Input: part model. Units: mm. Frame: model coordinates. Face numbers are marked on the shaded views. A direction names the side the tool comes from. Round coordinates to 2 decimals unless told otherwise and drop trailing zeros. Order: outer loops, then holes, each group sorted by start corner. A loop starts at its lowest first (then second) coordinate and runs counter-clockwise, first axis right, second up. Notation, with made-up numbers: (-8.75, -25) - (5.25, -25) arc R30 cw to (5.25, 7) - close; hole circle Ø5 at (87.5, 54.25). An arc over 180 degrees is marked (long way). One line per item, written item: value. Start each with the question number.
from build123d import *

# Parameters (mm, degrees)
SKETCH_1_W           = 25
SKETCH_1_H           = 21
EXTRUDE_2_DEPTH      = 34
SKETCH_2_W           = 10
SKETCH_2_H           = 9
SKETCH_2_R           = 1
CUT_EXTRUDE_4_DEPTH  = 60
SKETCH_3_R           = 1
SKETCH_3_W           = 13
SKETCH_3_H           = 38
CUT_EXTRUDE_2_DEPTH  = 44.488504228
SKETCH_6_W           = 3.5
SKETCH_6_H           = 7
CUT_EXTRUDE_5_DEPTH  = 9
SKETCH_11_W          = 3.5
SKETCH_11_H          = 7
CUT_EXTRUDE_9_DEPTH  = 9
SKETCH_7_R           = 1.25
CUT_EXTRUDE_6_DEPTH  = 42.871828238
SKETCH_9_W           = 25
SKETCH_9_H           = 10
CUT_EXTRUDE_7_DEPTH  = 2
SKETCH_10_W          = 25
SKETCH_10_H          = 10
CUT_EXTRUDE_8_DEPTH  = 2
CUT_EXTRUDE_START    = -6
SKETCH_12_W          = 13
SKETCH_12_H          = 68
CUT_EXTRUDE_10_DEPTH = 6
EXTRUDE_4_DEPTH      = 1.5
FILLET_R2_R          = 2
FILLET_R1_R          = 1


with BuildPart() as part:
    # 草图1 → 凸台-拉伸2 (new, symmetric)
    with BuildSketch(Plane(origin=(0, 0, 0), x_dir=(1, 0, 0), z_dir=(0, 1, 0))):
        Rectangle(SKETCH_1_W, SKETCH_1_H)
        Polygon((11.5, -3.5), (11.5, -6.5), (6.5, -6.5), (6, -6.5), (-6, -6.5), (-6.5, -6.5), (-11.5, -6.5), (-11.5, -3.5), (-6.5, -3.5), (-6.5, 3.5), (-11.5, 3.5), (-11.5, 6.5), (-6.5, 6.5), (-6, 6.5), (6, 6.5), (6.5, 6.5), (11.5, 6.5), (11.5, 3.5), (6.5, 3.5), (6.5, -3.5), align=None, mode=Mode.SUBTRACT)
    extrude(amount=EXTRUDE_2_DEPTH, both=True)

    # 草图2 → 切除-拉伸4 (cut)
    with BuildSketch(Plane(origin=(0, 0, -10.5), x_dir=(-1, 0, 0), z_dir=(0, 0, -1))):
        Polygon((9, -15), (9, 15), (6.25, 15), (6.25, 20), (3.25, 20), (3.25, 15), (-3.25, 15), (-3.25, 20), (-6.25, 20), (-6.25, 15), (-9, 15), (-9, -15), (-6.25, -15), (-6.25, -20), (-3.25, -20), (-3.25, -15), (3.25, -15), (3.25, -20), (6.25, -20), (6.25, -15), align=None)
        with Locations((0, -29.5)):
            Rectangle(SKETCH_2_W, SKETCH_2_H)
        with Locations((8.5, -22)):
            Circle(SKETCH_2_R)
        with Locations((-8.5, -22)):
            Circle(SKETCH_2_R)
        with Locations((-8.5, 22)):
            Circle(SKETCH_2_R)
        with Locations((8.5, 22)):
            Circle(SKETCH_2_R)
    extrude(amount=-CUT_EXTRUDE_4_DEPTH, mode=Mode.SUBTRACT)

    # 草图3 → 切除-拉伸2 (cut, through all)
    with BuildSketch(Plane(origin=(12.5, 0, 0), x_dir=(0, 0, -1), z_dir=(1, 0, 0))):
        with Locations((8.5, -17)):
            Circle(SKETCH_3_R)
        with Locations(Location((8.5, 17, 0), (0, 0, 180))):
            Circle(SKETCH_3_R)
        with Locations((-8.5, 17)):
            Circle(SKETCH_3_R)
        with Locations((-8.5, -17)):
            Circle(SKETCH_3_R)
        Rectangle(SKETCH_3_W, SKETCH_3_H)
    extrude(amount=-CUT_EXTRUDE_2_DEPTH, mode=Mode.SUBTRACT)

    # 草图6 → 切除-拉伸5 (cut)
    with BuildSketch(Plane.XZ.offset(34)):
        with Locations((8.25, 0)):
            Rectangle(SKETCH_6_W, SKETCH_6_H)
        with Locations((-8.25, 0)):
            Rectangle(SKETCH_6_W, SKETCH_6_H)
    extrude(amount=-CUT_EXTRUDE_5_DEPTH, mode=Mode.SUBTRACT)

    # 草图11 → 切除-拉伸9 (cut)
    with BuildSketch(Plane(origin=(0, 34, 0), x_dir=(1, 0, 0), z_dir=(0, 1, 0))):
        with Locations((-8.25, 0)):
            Rectangle(SKETCH_11_W, SKETCH_11_H)
        with Locations((8.25, 0)):
            Rectangle(SKETCH_11_W, SKETCH_11_H)
    extrude(amount=-CUT_EXTRUDE_9_DEPTH, mode=Mode.SUBTRACT)

    # 草图7 → 切除-拉伸6 (cut, through all)
    with BuildSketch(Plane(origin=(0, 0, -10.5), x_dir=(-1, 0, 0), z_dir=(0, 0, -1))):
        with Locations((8, -29)):
            Circle(SKETCH_7_R)
        with Locations(Location((-8, -29, 0), (0, 0, 180))):
            Circle(SKETCH_7_R)
        with Locations((-8, 29)):
            Circle(SKETCH_7_R)
        with Locations(Location((8, 29, 0), (0, 0, 180))):
            Circle(SKETCH_7_R)
    extrude(amount=-CUT_EXTRUDE_6_DEPTH, mode=Mode.SUBTRACT)

    # 草图9 → 切除-拉伸7 (cut)
    with BuildSketch(Plane(origin=(0, 0, -10.5), x_dir=(-1, 0, 0), z_dir=(0, 0, -1))):
        with Locations((0, 29)):
            Rectangle(SKETCH_9_W, SKETCH_9_H)
    extrude(amount=-CUT_EXTRUDE_7_DEPTH, mode=Mode.SUBTRACT)

    # 草图10 → 切除-拉伸8 (cut)
    with BuildSketch(Plane.XY.offset(10.5)):
        with Locations((0, 29)):
            Rectangle(SKETCH_10_W, SKETCH_10_H)
    extrude(amount=-CUT_EXTRUDE_8_DEPTH, mode=Mode.SUBTRACT)

    # 草图12 → 切除-拉伸10 (cut)
    with BuildSketch(Plane(origin=(12.5, 0, 0), x_dir=(0, 0, -1), z_dir=(1, 0, 0)).offset(CUT_EXTRUDE_START)):
        Rectangle(SKETCH_12_W, SKETCH_12_H)
    extrude(amount=CUT_EXTRUDE_10_DEPTH, mode=Mode.SUBTRACT)

    # 草图13 → 凸台-拉伸4 (add)
    with BuildSketch(Plane(origin=(-11.5, 0, 0), x_dir=(0, 0, -1), z_dir=(1, 0, 0))):
        with BuildLine():
            Line((-6.5, -34), (-3.5, -34))
            Line((-3.5, -34), (-3.5, -23.5))
            ThreePointArc((-3.5, -23.5), (-5, -25), (-6.5, -23.5))
            Line((-6.5, -23.5), (-6.5, -34))
        make_face()
        with BuildLine():
            Line((3.5, -34), (3.5, -23.5))
            ThreePointArc((3.5, -23.5), (5, -25), (6.5, -23.5))
            Line((6.5, -23.5), (6.5, -34))
            Line((6.5, -34), (3.5, -34))
        make_face()
        with BuildLine():
            Line((-3.5, 34), (-3.5, 23.5))
            ThreePointArc((-3.5, 23.5), (-5, 25), (-6.5, 23.5))
            Line((-6.5, 23.5), (-6.5, 34))
            Line((-6.5, 34), (-3.5, 34))
        make_face()
        with BuildLine():
            Line((6.5, 34), (6.5, 23.5))
            ThreePointArc((6.5, 23.5), (5, 25), (3.5, 23.5))
            Line((3.5, 23.5), (3.5, 34))
            Line((3.5, 34), (6.5, 34))
        make_face()
    extrude(amount=EXTRUDE_4_DEPTH)

    # R2
    fillet_r2_edges = [part.edges().sort_by_distance(p)[0] for p in [
        (5, -25, 8.5),
        (5, -25, -8.5),
        (-5, -25, 8.5),
        (-5, -25, -8.5),
        (9, -15, 8.5),
        (9, -15, -8.5),
        (9, 15, 8.5),
        (9, 15, -8.5),
        (-9, 15, 8.5),
        (-9, 15, -8.5),
        (-9, -15, 8.5),
        (-9, -15, -8.5),
        (-12, -19, 6.5),
        (-12, 19, -6.5),
        (-12, 19, 6.5),
        (-12, -19, -6.5),
    ]]
    fillet(fillet_r2_edges, radius=FILLET_R2_R)

    # R1
    fillet_r1_edges = [part.edges().sort_by_distance(p)[0] for p in [
        (-3.25, -20, 8.5),
        (-3.25, -20, -8.5),
        (-6.25, -20, 8.5),
        (-6.25, -20, -8.5),
        (3.25, -20, 8.5),
        (3.25, -20, -8.5),
        (6.25, -20, 8.5),
        (6.25, -20, -8.5),
        (6.25, 20, 8.5),
        (6.25, 20, -8.5),
        (3.25, 20, 8.5),
        (3.25, 20, -8.5),
        (-3.25, 20, 8.5),
        (-3.25, 20, -8.5),
        (-6.25, 20, 8.5),
        (-6.25, 20, -8.5),
    ]]
    fillet(fillet_r1_edges, radius=FILLET_R1_R)


solid = part.part
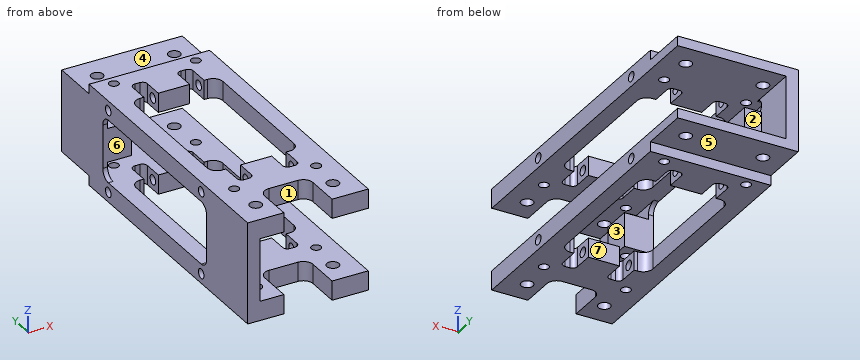
Item 1: First-contact query: pin 1 Ø5 at (y, z) = (-29, 3) entering from +X; pin 2 Ø0.5 at (x, z) = (4.5, 8) entering from -Y; pin 3 Ø4.5 at (x, z) = (1.5, -8.5) entering from -Y. Flat tips, straight axial feed; report the tip coordinate or a pass-through.
Item 2: Section query B-B on y = -29. Give the number of separate pieces and of enclosed holes in the cut face, and give its area (4 significant figures).
Item 3: Section query C-C on z = 2.75. Return loops of the section in (x, y), and give its area (3 significant figures).
Item 4: Reachability of the marked faces 4, 5, 6 and 7 from +Z, -Z, +X, -X, +Y, -Y: full face, straight path, thin tool, end or side. Return the list, or none.
Item 5: Line query: L1, parallel to Z at x = -8, y = 15; L2, parallel to X at y = -2, z = -7.25; L3, parallel to Y at x = -3, z = -9. Output: solid intervals per line, ascending.
Item 6: Section query D-D on y = -6.5. Return loops of the section in (x, z), and give its area (3 significant figures).
Item 7: Section query A-A on x = 10.25. Return loops of the section in (y, z).
Item 8: Pull-direction query (X, two-part tool) for the marked faces 1, 2 and 3; classes: released by +X, released by -X, zero draft, split by the parting line, or undercut.
Geometry results:
1. pin 1: stops at x = -10
1. pin 2: stops at y = -26.03
1. pin 3: stops at y = -25.15
2. separate pieces: 7
2. enclosed holes: 0
2. area: 112.5 mm^2
3. outline: (-12.5, -34) - (-10, -34) - (-10, -25) - (-6.5, -25) - (-6.5, -19) - (-12.5, -19) - close; (-12.5, 19) - (-6.5, 19) - (-6.5, 25) - (-10, 25) - (-10, 34) - (-12.5, 34) - close; hole circle Ø2 at (-8.5, -22); hole circle Ø2 at (-8.5, 22)
3. area: 111 mm^2
4. face 4: +Z, +X, -X, +Y
4. face 5: -Z, +X, -X, +Y
4. face 6: +X, -X
4. face 7: +Z, -Z
5. L1: z = -10.5 to -6.5, 6.5 to 10.5
5. L2: x = -12.5 to -9, 9 to 12.5
5. L3: y = -25 to -17.87, -16.13 to -15, 15 to 16.13, 17.87 to 24
6. outline: (-12.5, -10.5) - (-9, -10.5) - (-9, -6.5) - (-12.5, -6.5) - close; (-12.5, 6.5) - (-9, 6.5) - (-9, 10.5) - (-12.5, 10.5) - close; (9, -10.5) - (12.5, -10.5) - (12.5, -6.5) - (9, -6.5) - close; (9, 6.5) - (12.5, 6.5) - (12.5, 10.5) - (9, 10.5) - close
6. area: 56.0 mm^2
7. outline: (-34, -10.5) - (24, -10.5) - (24, -8.5) - (34, -8.5) - (34, -6.5) - (-34, -6.5) - close; (-34, 6.5) - (34, 6.5) - (34, 8.5) - (24, 8.5) - (24, 10.5) - (-34, 10.5) - close; hole circle Ø2 at (-17, -8.5); hole circle Ø2 at (-17, 8.5); hole circle Ø2 at (17, -8.5); hole circle Ø2 at (17, 8.5)
8. face 1: undercut
8. face 2: zero draft
8. face 3: released by +X
